Geometry: final body of the model. Coordinates: model frame, mm. Round coordinates to 2 decimals unless told otherwise and drop trailing zeros. Loops run counter-clockwise (first coordinate to the right, second up) from the corner with the lowest first, then second, coordinate; pieces in that order, holes last. Notation, with made-up numbers: (0, 41) - (28, 41) arc R13 cw to (28, 63) - close; hole circle Ø10 at (13, 86). An arc over 180 degrees is marked (long way). Return JSON: item names as keys, results as strings. Group by question number.
1. Section C-C on x = 29. Return loops of the section in (y, z) (3 decimals).
2. Material intervals for probe 1 along X at (y, z) = (1.1, -84); probe 2 along X at (y, z) = (2.15, -6.35), sorted ascending.
3. Section D-D on y = 1.1. Count the separate pieces of the cut face and the enclosed holes in it, and give its area (3 significant figures).
4. Section A-A on z = -6.35. Return loops of the section in (x, y) (3 decimals), and give its area (3 significant figures).
5. Section B-B on x = 0. Return loops of the section in (y, z) (3 decimals), and give its area (3 significant figures).
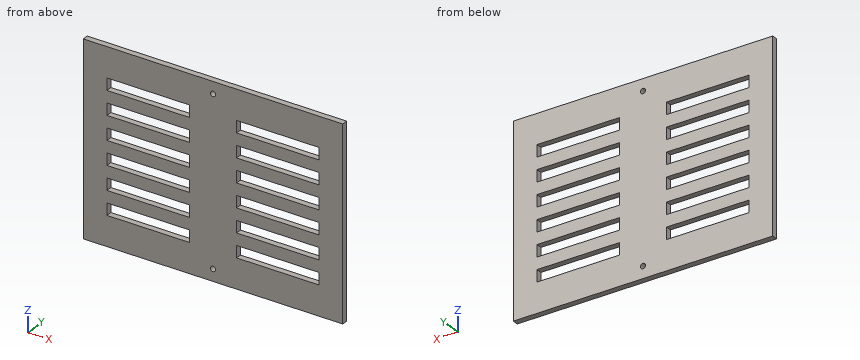
from build123d import *

# Parameters (mm, degrees)
SKETCH1_W           = 139.5984
SKETCH1_H           = 101.6
BOSS_EXTRUDE1_DEPTH = 3.175
SKETCH2_R           = 1.3843
SKETCH2_W           = 44.3992
SKETCH2_H           = 6.35
CUT_EXTRUDE1_DEPTH  = 3.175


with BuildPart() as part:
    # Sketch1 → Boss-Extrude1 (new body)
    with BuildSketch(Plane(origin=(0, 0, 0), x_dir=(1, 0, 0), z_dir=(0, 1, 0))):
        with Locations((0, 50.8)):
            Rectangle(SKETCH1_W, SKETCH1_H)
    extrude(amount=BOSS_EXTRUDE1_DEPTH)

    # Sketch2 → Cut-Extrude1 (cut)
    with BuildSketch(Plane(origin=(0, 3.175, 0), x_dir=(1, 0, 0), z_dir=(0, 1, 0))):
        with Locations(Location((0, 6.35, 0), (0, 0, 270))):
            Circle(SKETCH2_R)
        with Locations(Location((0, 95.25, 0), (0, 0, 270))):
            Circle(SKETCH2_R)
        with Locations((-34.8996, 82.55)):
            Rectangle(SKETCH2_W, SKETCH2_H)
        with Locations((-34.8996, 69.85)):
            Rectangle(SKETCH2_W, SKETCH2_H)
        with Locations((-34.8996, 57.15)):
            Rectangle(SKETCH2_W, SKETCH2_H)
        with Locations((-34.8996, 44.45)):
            Rectangle(SKETCH2_W, SKETCH2_H)
        with Locations((-34.8996, 31.75)):
            Rectangle(SKETCH2_W, SKETCH2_H)
        with Locations((-34.8996, 19.05)):
            Rectangle(SKETCH2_W, SKETCH2_H)
        with Locations((34.8996, 82.55)):
            Rectangle(SKETCH2_W, SKETCH2_H)
        with Locations((34.8996, 69.85)):
            Rectangle(SKETCH2_W, SKETCH2_H)
        with Locations((34.8996, 57.15)):
            Rectangle(SKETCH2_W, SKETCH2_H)
        with Locations((34.8996, 44.45)):
            Rectangle(SKETCH2_W, SKETCH2_H)
        with Locations((34.8996, 31.75)):
            Rectangle(SKETCH2_W, SKETCH2_H)
        with Locations((34.8996, 19.05)):
            Rectangle(SKETCH2_W, SKETCH2_H)
    extrude(amount=-CUT_EXTRUDE1_DEPTH, mode=Mode.SUBTRACT)


solid = part.part
Taken from the geometry:
{
 "1": {"outline": "(0, -101.6) - (3.175, -101.6) - (3.175, -85.725) - (0, -85.725) - close; (0, -79.375) - (3.175, -79.375) - (3.175, -73.025) - (0, -73.025) - close; (0, -66.675) - (3.175, -66.675) - (3.175, -60.325) - (0, -60.325) - close; (0, -53.975) - (3.175, -53.975) - (3.175, -47.625) - (0, -47.625) - close; (0, -41.275) - (3.175, -41.275) - (3.175, -34.925) - (0, -34.925) - close; (0, -28.575) - (3.175, -28.575) - (3.175, -22.225) - (0, -22.225) - close; (0, -15.875) - (3.175, -15.875) - (3.175, 0) - (0, 0) - close"},
 "2": {"probe 1": "-69.8 to -57.1, -12.7 to 12.7, 57.1 to 69.8", "probe 2": "-69.8 to -1.38, 1.38 to 69.8"},
 "3": {"separate pieces": "1", "enclosed holes": "14", "area": "10,800 mm2"},
 "4": {"outline": "(-69.799, 0) - (-1.384, 0) - (-1.384, 3.175) - (-69.799, 3.175) - close; (1.384, 0) - (69.799, 0) - (69.799, 3.175) - (1.384, 3.175) - close", "area": "434 mm2"},
 "5": {"outline": "(0, -101.6) - (3.175, -101.6) - (3.175, -96.634) - (0, -96.634) - close; (0, -93.866) - (3.175, -93.866) - (3.175, -7.734) - (0, -7.734) - close; (0, -4.966) - (3.175, -4.966) - (3.175, 0) - (0, 0) - close", "area": "305 mm2"}
}
